Can you work these out from the drawing? Everything is in mm from the part's minimum corner. A direction names the side the tool comes from. Round coordinates to 2 decimals unless told otherwise and drop trailing zeros. Loops run counter-clockwise (first coordinate to the right, second up) from the corner with the lowest first, then second, coordinate; pieces in that order, holes last. Notation, with made-up numbers: (-4.5, 22) -> (11.5, 22) arc R28 cw to (11.5, 53) -> close; hole circle Ø9 at (-10.75, 81.5). An arc over 180 degrees is marked (long way). Answer as a JSON object with one key per item and string values.
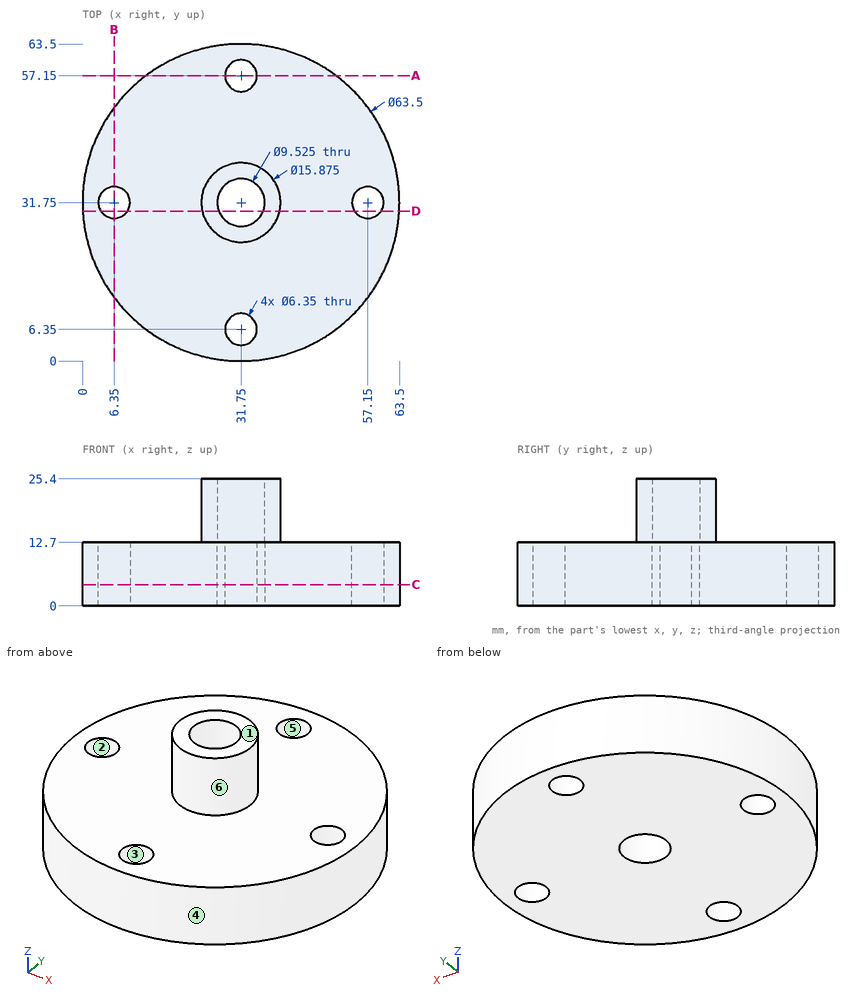
Q1. I want a section at D-D, the plane y = 30. Write out the boundary of the cut face in (x, z).
Determined:
{"outline": "(0.05, 0) -> (3.7, 0) -> (3.7, 12.7) -> (0.05, 12.7) -> close; (9, 0) -> (27.32, 0) -> (27.32, 25.4) -> (24.01, 25.4) -> (24.01, 12.7) -> (9, 12.7) -> close; (36.18, 0) -> (54.5, 0) -> (54.5, 12.7) -> (39.49, 12.7) -> (39.49, 25.4) -> (36.18, 25.4) -> close; (59.8, 0) -> (63.45, 0) -> (63.45, 12.7) -> (59.8, 12.7) -> close"}
Q2. We'd pull the mould along X, two halves only. Please class the marked faces 1, 2, 3 and 4: pulls with the +X half, pulls with the -X half, needs draft (parallel to the pull), parting line crosses it, or undercut.
Determined:
{"face 1": "needs draft", "face 2": "undercut", "face 3": "undercut", "face 4": "parting line crosses it"}
Q3. I want a section at C-C, the plane z = 4.25. Give the number of separate pieces and of enclosed holes in the cut face, then the cut area to 3 significant figures.
Determined:
{"separate pieces": "1", "enclosed holes": "5", "area": "2,970 mm²"}
Q4. I want a section at A-A, the plane y = 57.15. Write out the boundary of the cut face in (x, z) (3 decimals), then the cut area to 3 significant figures.
Determined:
{"outline": "(12.7, 0) -> (28.575, 0) -> (28.575, 12.7) -> (12.7, 12.7) -> close; (34.925, 0) -> (50.8, 0) -> (50.8, 12.7) -> (34.925, 12.7) -> close", "area": "403 mm²"}
Q5. If I drill on L1, parallel to Y at x = 31.75, z = 5.5 (1 decimal); L2, parallel to X at y = 30, z = 1.75; L3, parallel to Z at x = 43, y = 6.5, over which ranges is the centre line in solid material (lowest first)? Write a range as [from, to].
Determined:
{"L1": "[0, 3.2], [9.5, 27], [36.5, 54], [60.3, 63.5]", "L2": "[0.05, 3.7], [9, 27.32], [36.18, 54.5], [59.8, 63.45]", "L3": "[0, 12.7]"}
Q6. On a 3-axis mill with a long thin cutter (end or side, diameter ignored), from which of +Z, -Z, +X, -X, +Y, -Y can I reach the whole of each face in a straight line? I mean the marked faces 5 and 6. Say none if no direction works.
Determined:
{"face 5": "+Z, -Z", "face 6": "+Z"}
Q7. I'm going to push flat-ended pins straight in: pin 1 (8.5 mm diameter, centred on x = 31.75, y = 57.15, fed in from +Z); pin 2 (5 mm diameter, centred on x = 35, z = 9, fed in from -Y); pin 3 (1 mm diameter, centred on y = 53.5, z = 9.5, fed in from -X). Where does each tip first touch, or does it pass through?
Determined:
{"pin 1": "z = 12.7", "pin 2": "y = 0.01", "pin 3": "x = 8.16"}
